Answer from the drawing. Dimensions are ordinates in mm from the lowest x, y and z of the part. Coordinates: 2 decimals unless noted, no trailing zeros. Order: outer loops, then holes, each group sorted by start corner. A loop starts at its lowest first (then second) coordinate and runs counter-clockwise, first axis right, second up. Notation, with made-up numbers: (-18.75, 44.5) -> (27.25, 44.5) arc R18 cw to (27.25, 70.5) -> close; hole circle Ø6 at (31.25, 67.5). An arc over 180 degrees is marked (long way). Answer in a Markdown table with one row per item.
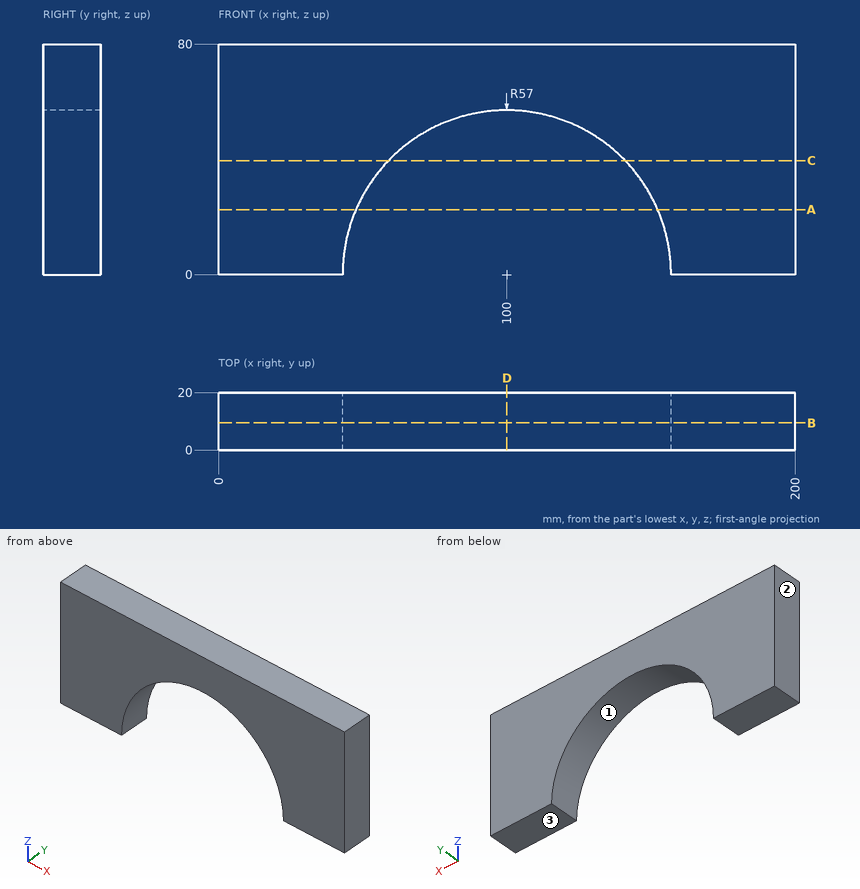
(1) A cutting plane is placed at B-B, the plane y = 9.5. Determine the outline of the cut face in (x, z).
Check values:
| item | result |
|---|---|
| outline | (0, 0) -> (43, 0) arc R57 cw to (157, 0) -> (200, 0) -> (200, 80) -> (0, 80) -> close |
(2) A cutting plane is placed at A-A, the plane z = 22.5. Determine the outline of the cut face in (x, y), then the cut area to 3 significant figures.
Check values:
| item | result |
|---|---|
| outline | (0, 0) -> (47.63, 0) -> (47.63, 20) -> (0, 20) -> close; (152.37, 0) -> (200, 0) -> (200, 20) -> (152.37, 20) -> close |
| area | 1,910 mm² |
(3) A cutting plane is placed at D-D, the plane x = 100. Determine the outline of the cut face in (y, z).
Check values:
| item | result |
|---|---|
| outline | (0, 57) -> (20, 57) -> (20, 80) -> (0, 80) -> close |
(4) For a pull along X with two mould halves and no side action, classify the marked faces 1, 2 and 3 as released by +X, released by -X, zero draft, split by the parting line, or undercut.
Check values:
| item | result |
|---|---|
| face 1 | undercut |
| face 2 | released by -X |
| face 3 | zero draft |
(5) A cutting plane is placed at C-C, the plane z = 39.5. Determine the outline of the cut face in (x, y), then the cut area to 3 significant figures.
Check values:
| item | result |
|---|---|
| outline | (0, 0) -> (58.91, 0) -> (58.91, 20) -> (0, 20) -> close; (141.09, 0) -> (200, 0) -> (200, 20) -> (141.09, 20) -> close |
| area | 2,360 mm² |
(6) Find the intervals of material crossed by line 1 along X through (y, z) = (5.25, 20); line 2 along X through (y, z) = (5.75, 44.5); line 3 along Z through (x, y) = (100.5, 6.25), in increasing order. Write a range as from..to.
Check values:
| item | result |
|---|---|
| line 1 | 0..46.62, 153.38..200 |
| line 2 | 0..64.38, 135.62..200 |
| line 3 | 57..80 |
